Geometry: final body of the model. Coordinates: model frame, mm. A direction names the side the tool comes from. Coordinates: 2 decimals unless noted, no trailing zeros. Loops run counter-clockwise (first coordinate to the right, second up) from the corner with the lowest first, then second, coordinate; pieces in that order, holes last. Notation, with made-up numbers: (-19.5, 77) -> (6.5, 77) arc R37 cw to (6.5, 115) -> close; hole circle Ø6 at (-23.5, 25.25). An arc over 180 degrees is marked (long way). One line per item, written item: value. Start each with the question number.
Item 1: Section query A-A on y = 0. Return loops of the section in (x, z).
Item 2: Section query D-D on x = -16. Return loops of the section in (y, z).
Item 3: Section query B-B on z = -6.5. Return loops of the section in (x, y).
Item 4: Section query C-C on x = 0. Return loops of the section in (y, z).
Item 5: Contact query for flat-ended pins moving along their axis: pin 1 Ø4 at (x, y) = (-9.9, 9.9) entering from -Z; pin 2 Ø2.5 at (x, y) = (9.9, -9.9) entering from +Z; pin 3 Ø1.5 at (x, z) = (12.5, -12) entering from +Y. Output: stop coordinate, or through.
Item 6: Set-up query: faces 1 (the flat face through (0, -21.5, -19)), 2 (the cylindrical face through (-14.727, -22.979, -4.418)). Return all of +Z, -Z, +X, -X, +Y, -Y with unobstructed straight access to the full face (end or side cutting, diameter ignored); none if empty.
Item 7: Mould query, pull axis X, two halves, no side actions, for faces 3 (the flat face through (-20, -23, -8)), 4 (the cylindrical face through (11.08, 8.82, 1.48)), 5 (the flat face through (20, -23, -8)). Classes: +X half, -X half, draft (parallel to the pull), parting line (faces both ways), or undercut.
Item 8: Ray query, probe 1 along Z at (x, y) = (15, -23.8); probe 2 along Y at (x, z) = (-11, -30); probe 3 along Z at (x, y) = (15.5, -18). Return the intervals inside material, ascending. Write a range as from..to.
from build123d import *

# Parameters (mm, degrees)
SKETCH_1_W          = 40
SKETCH_1_H          = 45
SKETCH_1_R          = 11.1
SKETCH_1_R_2        = 1.6
EXTRUDE_1_DEPTH     = 3
SKETCH_2_W          = 40
SKETCH_2_H          = 3
EXTRUDE_2_DEPTH     = 41.5
SKETCH_3_R          = 2.1
CUT_EXTRUDE_1_DEPTH = 61.384186672
FILLET_1_R          = 10
FILLET_3_R          = 3
FILLET_4_R          = 1


with BuildPart() as part:
    # 草图1 → 凸台-拉伸1 (new body)
    with BuildSketch(Plane.XY):
        with Locations((0, -2)):
            Rectangle(SKETCH_1_W, SKETCH_1_H)
        Circle(SKETCH_1_R, mode=Mode.SUBTRACT)
        with Locations((-9.899494937, 9.899494937)):
            Circle(SKETCH_1_R_2, mode=Mode.SUBTRACT)
        with Locations(Location((9.899494937, 9.899494937, 0), (0, 0, 180))):
            Circle(SKETCH_1_R_2, mode=Mode.SUBTRACT)
        with Locations(Location((-9.899494937, -9.899494937, 0), (0, 0, 180))):
            Circle(SKETCH_1_R_2, mode=Mode.SUBTRACT)
        with Locations((9.899494937, -9.899494937)):
            Circle(SKETCH_1_R_2, mode=Mode.SUBTRACT)
    extrude(amount=EXTRUDE_1_DEPTH)

    # 草图2 → 凸台-拉伸2 (add)
    with BuildSketch(Plane.XY.offset(3)):
        with Locations((0, -23)):
            Rectangle(SKETCH_2_W, SKETCH_2_H)
    extrude(amount=-EXTRUDE_2_DEPTH)

    # 草图3 → 切除-拉伸1 (cut, through all)
    with BuildSketch(Plane(origin=(0, -21.5, 0), x_dir=(1, 0, 0), z_dir=(0, 1, 0))):
        with Locations(Location((-15, 31, 0), (0, 0, 180))):
            Circle(SKETCH_3_R)
        with Locations((15, 31)):
            Circle(SKETCH_3_R)
        with Locations((15, 6.5)):
            Circle(SKETCH_3_R)
        with Locations(Location((-15, 6.5, 0), (0, 0, 180))):
            Circle(SKETCH_3_R)
    extrude(amount=-CUT_EXTRUDE_1_DEPTH, mode=Mode.SUBTRACT)

    # 圆角1
    fillet_1_edges = [part.edges().sort_by_distance(p)[0] for p in [
        (-20, 20.5, 1.5),
        (20, 20.5, 1.5),
    ]]
    fillet(fillet_1_edges, radius=FILLET_1_R)

    # 圆角3
    fillet_3_edges = [part.edges().sort_by_distance(p)[0] for p in [
        (0, -24.5, 3),
    ]]
    fillet(fillet_3_edges, radius=FILLET_3_R)

    # 圆角4
    fillet_4_edges = [part.edges().sort_by_distance(p)[0] for p in [
        (0, -21.5, 0),
    ]]
    fillet(fillet_4_edges, radius=FILLET_4_R)


solid = part.part
Reply:
1. outline: (-20, 0) -> (-11.1, 0) -> (-11.1, 3) -> (-20, 3) -> close; (11.1, 0) -> (20, 0) -> (20, 3) -> (11.1, 3) -> close
2. outline: (-24.5, -38.5) -> (-21.5, -38.5) -> (-21.5, -32.85) -> (-24.5, -32.85) -> close; (-24.5, -29.15) -> (-21.5, -29.15) -> (-21.5, -8.35) -> (-24.5, -8.35) -> close; (-24.5, -4.65) -> (-21.5, -4.65) -> (-21.5, -1) arc R1 cw to (-20.5, 0) -> (18.5, 0) -> (18.5, 3) -> (-21.5, 3) arc R3 ccw to (-24.5, 0) -> close
3. outline: (-20, -24.5) -> (-17.1, -24.5) -> (-17.1, -21.5) -> (-20, -21.5) -> close; (-12.9, -24.5) -> (12.9, -24.5) -> (12.9, -21.5) -> (-12.9, -21.5) -> close; (17.1, -24.5) -> (20, -24.5) -> (20, -21.5) -> (17.1, -21.5) -> close
4. outline: (-24.5, -38.5) -> (-21.5, -38.5) -> (-21.5, -1) arc R1 cw to (-20.5, 0) -> (-11.1, 0) -> (-11.1, 3) -> (-21.5, 3) arc R3 ccw to (-24.5, 0) -> close; (11.1, 0) -> (20.5, 0) -> (20.5, 3) -> (11.1, 3) -> close
5. pin 1: stops at z = 0
5. pin 2: passes through
5. pin 3: stops at y = -21.5
6. face 1: -Z, +X, -X, +Y
6. face 2: +Y, -Y
7. face 3: -X half
7. face 4: undercut
7. face 5: +X half
8. probe 1: z = -38.5..-33.1, -28.9..-8.6, -4.4..1.93
8. probe 2: y = -24.5..-21.5
8. probe 3: z = 0..3
